Model file for the job. Use its own axes, mm. A direction names the side the tool comes from. Coordinates: 2 decimals unless noted, no trailing zeros. Loops run counter-clockwise (first coordinate to the right, second up) from the corner with the lowest first, then second, coordinate; pieces in that order, holes last.
from build123d import *

# Parameters (mm, degrees)
SKETCH1_W           = 24
SKETCH1_H           = 13
BOSS_EXTRUDE1_DEPTH = 15
SKETCH2_W           = 20.15
SKETCH2_H           = 1.75
CUT_EXTRUDE1_DEPTH  = 15
FILLET1_R           = 2
CHAMFER2_SIZE       = 1
CHAMFER2_SIZE2      = 2.747477419
FILLET2_R           = 0.5
CUT_EXTRUDE4_DEPTH  = 11
SKETCH5_W           = 26.855674208
SKETCH5_H           = 19.307728506
CUT_EXTRUDE5_DEPTH  = 8
CUT_EXTRUDE6_DEPTH  = 11
SKETCH7_W           = 29.982721697
SKETCH7_H           = 21.559004648
CUT_EXTRUDE7_DEPTH  = 3
CHAMFER3_SIZE       = 2
FILLET3_R           = 0.4
FILLET4_R           = 0.2
SKETCH8_W           = 7
SKETCH8_H           = 2.8
CUT_EXTRUDE8_DEPTH  = 21.808652047
FILLET5_R           = 0.5


with BuildPart() as part:
    # Sketch1 → Boss-Extrude1 (new body)
    with BuildSketch(Plane(origin=(0, 0, 0), x_dir=(1, 0, 0), z_dir=(0, 1, 0))):
        Rectangle(SKETCH1_W, SKETCH1_H)
    extrude(amount=BOSS_EXTRUDE1_DEPTH)

    # Sketch2 → Cut-Extrude1 (cut)
    with BuildSketch(Plane.XY.offset(6.5)):
        with Locations((0, 7.575)):
            Rectangle(SKETCH2_W, SKETCH2_H)
    extrude(amount=-CUT_EXTRUDE1_DEPTH, mode=Mode.SUBTRACT)

    # Fillet1
    fillet1_edges = [part.edges().sort_by_distance(p)[0] for p in [
        (-12, 15, 0),
        (12, 15, 0),
        (-12, 0, 0),
        (12, 0, 0),
    ]]
    fillet(fillet1_edges, radius=FILLET1_R)

    # Chamfer2
    chamfer2_edges = [part.edges().sort_by_distance(p)[0] for p in [
        (0, 15, 6.5),
        (12, 7.5, 6.5),
        (0, 0, 6.5),
        (-12, 7.5, 6.5),
        (-11.414213562, 14.414213562, 6.5),
        (-11.414213562, 0.585786438, 6.5),
        (11.414213562, 0.585786438, 6.5),
        (11.414213562, 14.414213562, 6.5),
    ]]
    chamfer2_side = [part.faces().sort_by_distance(p)[0] for p in [
        (11.716980566, 7.5, 6.5),
    ]]
    chamfer(chamfer2_edges, length=CHAMFER2_SIZE, length2=CHAMFER2_SIZE2, reference=chamfer2_side[0])

    # Fillet2
    fillet2_edges = [part.edges().sort_by_distance(p)[0] for p in [
        (10.075, 7.575, 6.5),
        (0, 8.45, 6.5),
        (-10.075, 7.575, 6.5),
        (0, 6.7, 6.5),
    ]]
    fillet(fillet2_edges, radius=FILLET2_R)

    # Sketch4 → Cut-Extrude4 (cut)
    with BuildSketch(Plane(origin=(0, 0, -6.5), x_dir=(-1, 0, 0), z_dir=(0, 0, -1))):
        Polygon((-10.075, 8.45), (-8.575, 8.45), (-8.575, 11.891155889), (8.575, 11.891155889), (8.575, 8.45), (10.075, 8.45), (10.075, 6.7), (-10.075, 6.7), align=None)
    extrude(amount=-CUT_EXTRUDE4_DEPTH, mode=Mode.SUBTRACT)

    # Sketch5 → Cut-Extrude5 (cut)
    with BuildSketch(Plane(origin=(0, 0, -6.5), x_dir=(-1, 0, 0), z_dir=(0, 0, -1))):
        with Locations((-0.083402715, 7.762018115)):
            Rectangle(SKETCH5_W, SKETCH5_H)
        with BuildLine():
            Line((10, 14), (-10, 14))
            ThreePointArc((-10, 14), (-10.707106781, 13.707106781), (-11, 13))
            Line((-11, 13), (-11, 2))
            ThreePointArc((-11, 2), (-10.707106781, 1.292893219), (-10, 1))
            Line((-10, 1), (10, 1))
            ThreePointArc((10, 1), (10.707106781, 1.292893219), (11, 2))
            Line((11, 2), (11, 13))
            ThreePointArc((11, 13), (10.707106781, 13.707106781), (10, 14))
        make_face(mode=Mode.SUBTRACT)
    extrude(amount=-CUT_EXTRUDE5_DEPTH, mode=Mode.SUBTRACT)

    # Sketch6 → Cut-Extrude6 (cut)
    with BuildSketch(Plane(origin=(0, 0, -6.5), x_dir=(-1, 0, 0), z_dir=(0, 0, -1))):
        with BuildLine():
            Line((-9, 5.7), (9, 5.7))
            ThreePointArc((9, 5.7), (9.707106781, 5.407106781), (10, 4.7))
            Line((10, 4.7), (10, 3))
            ThreePointArc((10, 3), (9.707106781, 2.292893219), (9, 2))
            Line((9, 2), (-9, 2))
            ThreePointArc((-9, 2), (-9.707106781, 2.292893219), (-10, 3))
            Line((-10, 3), (-10, 4.7))
            ThreePointArc((-10, 4.7), (-9.707106781, 5.407106781), (-9, 5.7))
        make_face()
    extrude(amount=-CUT_EXTRUDE6_DEPTH, mode=Mode.SUBTRACT)

    # Sketch7 → Cut-Extrude7 (cut)
    with BuildSketch(Plane(origin=(0, 0, -6.5), x_dir=(-1, 0, 0), z_dir=(0, 0, -1))):
        with Locations((0.615824589, 7.279559508)):
            Rectangle(SKETCH7_W, SKETCH7_H)
    extrude(amount=-CUT_EXTRUDE7_DEPTH, mode=Mode.SUBTRACT)

    # Chamfer3
    chamfer3_edges = [part.edges().sort_by_distance(p)[0] for p in [
        (9.325, 8.45, -3.5),
        (-9.325, 8.45, -3.5),
    ]]
    chamfer(chamfer3_edges, length=CHAMFER3_SIZE)

    # Fillet3
    fillet3_edges = [part.edges().sort_by_distance(p)[0] for p in [
        (-10, 3.85, -3.5),
        (0, 14, -3.5),
        (-10.707106781, 13.707106781, -3.5),
        (-11, 7.5, -3.5),
        (-10.707106781, 1.292893219, -3.5),
        (0, 1, -3.5),
        (10.707106781, 1.292893219, -3.5),
        (11, 7.5, -3.5),
        (10.707106781, 13.707106781, -3.5),
        (0, 6.7, -3.5),
        (0, 11.891155889, -3.5),
        (-8.575, 11.170577944, -3.5),
        (-9.707106781, 2.292893219, -3.5),
        (0, 2, -3.5),
        (9.707106781, 2.292893219, -3.5),
        (10, 3.85, -3.5),
        (9.707106781, 5.407106781, -3.5),
        (0, 5.7, -3.5),
        (-9.707106781, 5.407106781, -3.5),
        (8.575, 11.170577944, -3.5),
        (-9.325, 10.45, -3.5),
        (9.325, 10.45, -3.5),
    ]]
    fillet(fillet3_edges, radius=FILLET3_R)

    # Fillet4
    fillet4_edges = [part.edges().sort_by_distance(p)[0] for p in [
        (-11.414213562, 14.414213562, 1.5),
        (0, 0, 1.5),
        (-12, 7.5, 1.5),
        (12, 7.5, 1.5),
        (11.414213562, 0.585786438, 1.5),
        (11.414213562, 14.414213562, 1.5),
        (0, 15, 1.5),
        (-11.414213562, 0.585786438, 1.5),
    ]]
    fillet(fillet4_edges, radius=FILLET4_R)

    # Sketch8 → Cut-Extrude8 (cut, through all)
    with BuildSketch(Plane(origin=(0, 0, 4.5), x_dir=(-1, 0, 0), z_dir=(0, 0, -1))):
        with Locations((0, 8.45)):
            Rectangle(SKETCH8_W, SKETCH8_H)
    extrude(amount=-CUT_EXTRUDE8_DEPTH, mode=Mode.SUBTRACT)

    # Fillet5
    fillet5_edges = [part.edges().sort_by_distance(p)[0] for p in [
        (-3.5, 8.45, 5.25),
        (-3.5, 9.4, 6.5),
        (-3.5, 9.85, 5.5),
        (3.5, 8.45, 5.25),
        (3.5, 9.4, 6.5),
        (-3.5, 8.596446609, 6.353553391),
        (3.5, 8.596446609, 6.353553391),
        (0, 9.85, 6.5),
        (3.5, 9.85, 5.5),
    ]]
    fillet(fillet5_edges, radius=FILLET5_R)


solid = part.part
Q1. Slice it at A-A (y = 7). List the corners of the cut face in (x, z) (3 decimals), and give its area (3 significant figures).
Answers:
outline: (-12, 1.7) arc R0.2 ccw to (-11.8, 1.5) - (-11, 1.5) - (-11, -3.1) arc R0.4 ccw to (-10.6, -3.5) - (-10.075, -3.5) - (-10.075, 6) arc R0.5 ccw to (-10.575, 6.5) - (-11, 6.5) - (-12, 3.753) - close; (10.075, -3.5) - (10.6, -3.5) arc R0.4 ccw to (11, -3.1) - (11, 1.5) - (11.8, 1.5) arc R0.2 ccw to (12, 1.7) - (12, 3.753) - (11, 6.5) - (10.575, 6.5) arc R0.5 ccw to (10.075, 6) - close
area: 25.6 mm2
Q2. Slice it at B-B (z = -2). List the corners of the cut face in (x, y) (3 decimals), and give its area (3 significant figures).
Answers:
outline: (-11, 2) arc R1 ccw to (-10, 1) - (10, 1) arc R1 ccw to (11, 2) - (11, 13) arc R1 ccw to (10, 14) - (-10, 14) arc R1 ccw to (-11, 13) - close; hole (-10.075, 6.7) - (10.075, 6.7) - (10.075, 8.95) - (8.575, 8.95) - (8.575, 11.891) - (-8.575, 11.891) - (-8.575, 8.95) - (-10.075, 8.95) - close; hole (-10, 3) arc R1 ccw to (-9, 2) - (9, 2) arc R1 ccw to (10, 3) - (10, 4.7) arc R1 ccw to (9, 5.7) - (-9, 5.7) arc R1 ccw to (-10, 4.7) - close
area: 116 mm2
Q3. Which spindle directions (+Z, -Z, +X, -X, +Y, -Y) get a long thin tool onto all of the face, cutting with end or side? Do faces 1 (the flat face through (0, 6.7, 2)), 2 (the flat face through (11, 8, -1)), 3 (the flat face through (10, 4, 1)). Say none if no direction does.
Answers:
face 1: +Z, -Z
face 2: -Z, +X, +Y, -Y
face 3: -Z
Q4. Flat gauge pins, fed straight in: P1, Ø4, axis at x = 3.5, y = 10.5, coming from the -Z side; P2, Ø2.5, axis at y = 8, z = -1.5, coming from the +X side; P3, Ø1, axis at x = 6.5, z = -0.5, coming from the +Y side; P4, Ø1, axis at x = 8, z = 0.5, coming from the -Y side. Where does each tip first touch, or does it go through?
Answers:
P1: stops at z = -3.5
P2: stops at x = 11
P3: stops at y = 14
P4: stops at y = 1
Q5. Mould opens along X. For faces 4 (the flat face through (12, 7, 3)), 5 (the flat face through (0.14, 0.493, 5.107)), 6 (the flat face through (9, 8.45, 4)) say: +X half, -X half, draft (parallel to the pull), parting line (faces both ways), or undercut.
Answers:
face 4: +X half
face 5: draft
face 6: undercut
Q6. Drill centre lines: line 1 (Y direction, x = 4, z = 3.25); line 2 (X direction, y = 7, z = -2) (3 decimals); line 3 (X direction, y = 8.5, z = 1.25) (3 decimals). Where is each one in solid material? Low to high.
Answers:
line 1: y = 0 to 2, 5.7 to 6.7, 11.89 to 15
line 2: x = -11 to -10.075, 10.075 to 11
line 3: x = -11 to -8.575, 8.575 to 11
